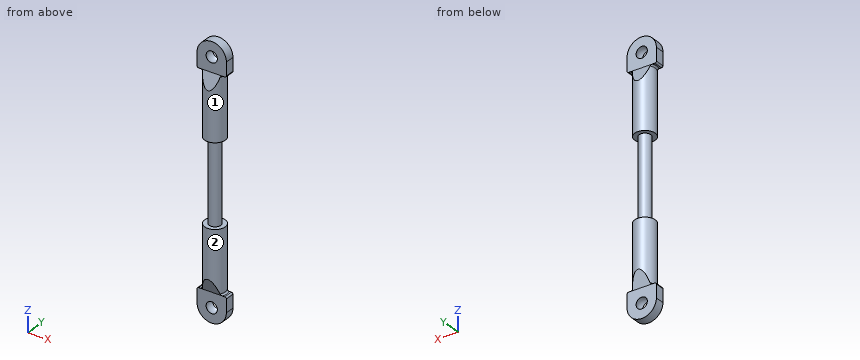
from build123d import *

# Parameters (mm, degrees)
SKETCH1_R                  = 2
SCREW_SECTION_DEPTH        = 14
SKETCH2_R                  = 3.5
BAR_SECTION_DEPTH          = 21.5
MOUNT_SECTION_DEPTH        = 1.6
BAR_TAPER_DEPTH            = 6
MOUNT_FILLET_R             = 0.5
MOUNT_FILLET_OF_MIRROR_2_R = 0.5


with BuildPart() as part:
    # Sketch1 → Screw Section (new body)
    with BuildSketch(Plane.XY):
        Circle(SKETCH1_R)
    screw_section = extrude(amount=SCREW_SECTION_DEPTH)

    # Sketch2 → Bar Section (add)
    with BuildSketch(Plane.XY.offset(14)):
        Circle(SKETCH2_R)
    bar_section = extrude(amount=BAR_SECTION_DEPTH)

    # Sketch3 → Mount Section (add, symmetric)
    with BuildSketch(Plane(origin=(0, 0, 0), x_dir=(1, 0, 0), z_dir=(0, 1, 0))):
        with BuildLine():
            Line((5, -35.5), (-5, -35.5))
            Line((-5, -35.5), (-5, -40.5))
            ThreePointArc((-5, -40.5), (0, -45.5), (5, -40.5))
            Line((5, -40.5), (5, -35.5))
        make_face()
    mount_section = extrude(amount=MOUNT_SECTION_DEPTH, both=True)

    # Sketch4 → Bar Taper (cut, symmetric)
    with BuildSketch(Plane(origin=(0, 0, 0), x_dir=(0, 0, -1), z_dir=(1, 0, 0))):
        Polygon((-30.5, -3.5), (-35.5, -1.6), (-35.5, -3.5), align=None)
        Polygon((-30.5, 3.5), (-35.5, 1.6), (-35.5, 3.5), align=None)
    bar_taper = extrude(amount=BAR_TAPER_DEPTH, both=True, mode=Mode.SUBTRACT)

    # Mount Fillet
    mount_fillet_edges = [part.edges().sort_by_distance(p)[0] for p in [
        (-5, 0, 35.5),
        (3.401842713, -0.823083322, 35.5),
        (-3.5, 0, 35.5),
        (5, 0, 35.5),
    ]]
    fillet(mount_fillet_edges, radius=MOUNT_FILLET_R)

    # Sketch6 → Ball Hole (revolve, cut)
    with BuildSketch(Plane(origin=(0, 0, 0), x_dir=(0, 0, -1), z_dir=(1, 0, 0))):
        with BuildLine():
            Line((-42.420937271, -1.6), (-40.5, -1.6))
            Line((-40.5, -1.6), (-40.5, 1.6))
            Line((-40.5, 1.6), (-42.420937271, 1.6))
            ThreePointArc((-42.420937271, 1.6), (-43, 0), (-42.420937271, -1.6))
        make_face()
    ball_hole = revolve(axis=Axis((0, -1.6, 40.5), (0, 1, 0)), mode=Mode.SUBTRACT)

    # Mirror 2: Screw Section, Bar Section, Mount Section, Bar Taper, Ball Hole across Front Plane
    add(screw_section.mirror(Plane.XY))
    add(bar_section.mirror(Plane.XY))
    add(mount_section.mirror(Plane.XY))
    add(bar_taper.mirror(Plane.XY), mode=Mode.SUBTRACT)
    add(ball_hole.mirror(Plane.XY), mode=Mode.SUBTRACT)

    # Mount Fillet of Mirror 2
    mount_fillet_of_mirror_2_edges = [part.edges().sort_by_distance(p)[0] for p in [
        (-5, 0, -35.5),
        (3.401842713, -0.823083322, -35.5),
        (-3.5, 0, -35.5),
        (5, 0, -35.5),
    ]]
    fillet(mount_fillet_of_mirror_2_edges, radius=MOUNT_FILLET_OF_MIRROR_2_R)


solid = part.part
Could you check a few things on this model? Use its own coordinates, in mm. Face numbers are marked on the shaded views. Give positions to 0.01 mm unless a question says otherwise; leave off trailing zeros. Loops run counter-clockwise (first coordinate to the right, second up) from the corner with the lowest first, then second, coordinate; pieces in that order, holes last. Notation, with made-up numbers: M 68.5,75 L 80.5,75 A30 ccw 80.5,97 Z; hole C 34.25,58.5 d2. An arc over 180 degrees is marked long. Answer as a JSON object with one key per item and string values.
Q1. If I drill on probe 1 along Z at (x, y) = (-1, -0.5); probe 2 along Z at (x, y) = (0.25, -1); probe 3 along Z at (x, y) = (3, -1.25), over which ranges is the centre line in solid material (lowest first)? Write a range as [from, to].
Values found:
{"probe 1": "z = [-45.4, -42.74], [-38.26, 38.26], [42.74, 45.4]", "probe 2": "z = [-45.49, -42.78], [-38.22, 38.22], [42.78, 45.49]", "probe 3": "z = [-44.5, -14], [14, 44.5]"}
Q2. Suppose I cut it at B-B, the plane x = 0. List the corners of the cut face in (y, z) for me.
Values found:
{"outline": "M -3.5,-30.5 L -1.6,-35.5 L -1.6,-38.58 A2.5 cw 1.6,-38.58 L 1.6,-35.5 L 3.5,-30.5 L 3.5,-14 L 2,-14 L 2,14 L 3.5,14 L 3.5,30.5 L 1.6,35.5 L 1.6,38.58 A2.5 cw -1.6,38.58 L -1.6,35.5 L -3.5,30.5 L -3.5,14 L -2,14 L -2,-14 L -3.5,-14 Z; M -1.6,-45.5 L 1.6,-45.5 L 1.6,-42.42 A2.5 cw -1.6,-42.42 Z; M -1.6,42.42 A2.5 cw 1.6,42.42 L 1.6,45.5 L -1.6,45.5 Z"}
Q3. For P1, Ø5, axis at x = 0, z = -43, coming from the +Y side; P2, Ø1.5, axis at x = -2, z = 20.5, coming from the +Y side; P3, Ø3, axis at x = 1.5, y = 2, coming from the +Z side; P4, Ø0.7, axis at x = 4, y = -0.5, coming from the +Z side, each with a flat end and sliding along its axis, tell me the tip position at first contact or that it passes through.
Values found:
{"P1": "stops at y = 1.6", "P2": "stops at y = 3.27", "P3": "stops at z = 45.5", "P4": "stops at z = 43.92"}
Q4. If we mould it in two halves opening along Z, with no side actions, what happens to the marked faces 1 and 2? For each: pulls with the +Z half, pulls with the -Z half, needs draft (parallel to the pull), parting line crosses it, or undercut.
Values found:
{"face 1": "undercut", "face 2": "undercut"}
Q5. Suppose I cut it at C-C, the plane z = 23. List the corners of the cut face in (x, y) for me, plus the area to 3 significant figures.
Values found:
{"outline": "C 0,0 d7", "area": "38.5 mm²"}
Q6. Suppose I cut it at A-A, the plane y = 0. State how many separate pieces and enclosed holes the cut face has, plus the area to 3 significant figures.
Values found:
{"separate pieces": "1", "enclosed holes": "2", "area": "552 mm²"}
Q7. Suppose I cut it at D-D, the plane z = 11.5. List the corners of the cut face in (x, y) for me.
Values found:
{"outline": "C 0,0 d4"}
